```python
from build123d import *

# Parameters (mm, degrees)
SKETCH_1_R      = 1.65
EXTRUDE_1_DEPTH = 2
EXTRUDE_3_DEPTH = 23.5
SKETCH_3_R      = 1.5
EXTRUDE_4_DEPTH = 2
FILLET_1_R      = 1


with BuildPart() as part:
    # 草图1 → 凸台-拉伸1 (new body)
    # profile 1 of 2: a face of its own
    with BuildSketch(Plane(origin=(0, 0, 0), x_dir=(1, 0, 0), z_dir=(0, 1, 0))):
        with BuildLine():
            ThreePointArc((0, 1.5), (0.439339828, 0.439339828), (1.5, 0))
            Line((1.5, 0), (26.5, 0))
            ThreePointArc((26.5, 0), (27.560660172, 0.439339828), (28, 1.5))
            Line((28, 1.5), (28, 14))
            ThreePointArc((28, 14), (27.225183212, 18.592878075), (24.986495855, 22.677379145))
            ThreePointArc((24.986495855, 22.677379145), (22.833273811, 22.833273811), (22.677379145, 24.986495855))
            ThreePointArc((22.677379145, 24.986495855), (18.592878075, 27.225183212), (14, 28))
            Line((14, 28), (1.5, 28))
            ThreePointArc((1.5, 28), (0.439339828, 27.560660172), (0, 26.5))
            Line((0, 26.5), (0, 1.5))
        make_face()
        with Locations(Location((4, 4, 0), (0, 0, 270))):
            Circle(SKETCH_1_R, mode=Mode.SUBTRACT)
        with Locations(Location((24, 4, 0), (0, 0, 270))):
            Circle(SKETCH_1_R, mode=Mode.SUBTRACT)
        with Locations(Location((4, 24, 0), (0, 0, 270))):
            Circle(SKETCH_1_R, mode=Mode.SUBTRACT)
        with BuildLine():
            Line((18.75, 8.8), (9.25, 8.8))
            ThreePointArc((9.25, 8.8), (8.189339828, 9.239339828), (7.75, 10.3))
            Line((7.75, 10.3), (7.75, 17.7))
            ThreePointArc((7.75, 17.7), (8.189339828, 18.760660172), (9.25, 19.2))
            Line((9.25, 19.2), (18.75, 19.2))
            ThreePointArc((18.75, 19.2), (19.810660172, 18.760660172), (20.25, 17.7))
            Line((20.25, 17.7), (20.25, 10.3))
            ThreePointArc((20.25, 10.3), (19.810660172, 9.239339828), (18.75, 8.8))
        make_face(mode=Mode.SUBTRACT)
    # profile 2 of 2: a face of its own
    with BuildSketch(Plane(origin=(0, 0, 0), x_dir=(1, 0, 0), z_dir=(0, 1, 0))):
        with BuildLine():
            ThreePointArc((22.677379145, 24.986495855), (22.833273811, 22.833273811), (24.986495855, 22.677379145))
            ThreePointArc((24.986495855, 22.677379145), (23.899494937, 23.899494937), (22.677379145, 24.986495855))
        make_face()
    extrude(amount=EXTRUDE_1_DEPTH)

    # 草图2 → 凸台-拉伸3 (add)
    with BuildSketch(Plane(origin=(0, 2, 0), x_dir=(1, 0, 0), z_dir=(0, 1, 0))):
        with BuildLine():
            Line((7.25, 21.2), (20.75, 21.2))
            ThreePointArc((20.75, 21.2), (21.810660172, 20.760660172), (22.25, 19.7))
            Line((22.25, 19.7), (22.25, 8.3))
            ThreePointArc((22.25, 8.3), (21.810660172, 7.239339828), (20.75, 6.8))
            Line((20.75, 6.8), (7.25, 6.8))
            ThreePointArc((7.25, 6.8), (6.189339828, 7.239339828), (5.75, 8.3))
            Line((5.75, 8.3), (5.75, 19.7))
            ThreePointArc((5.75, 19.7), (6.189339828, 20.760660172), (7.25, 21.2))
        make_face()
        with BuildLine():
            Line((9.25, 19.2), (18.75, 19.2))
            ThreePointArc((18.75, 19.2), (19.810660172, 18.760660172), (20.25, 17.7))
            Line((20.25, 17.7), (20.25, 10.3))
            ThreePointArc((20.25, 10.3), (19.810660172, 9.239339828), (18.75, 8.8))
            Line((18.75, 8.8), (9.25, 8.8))
            ThreePointArc((9.25, 8.8), (8.189339828, 9.239339828), (7.75, 10.3))
            Line((7.75, 10.3), (7.75, 17.7))
            ThreePointArc((7.75, 17.7), (8.189339828, 18.760660172), (9.25, 19.2))
        make_face(mode=Mode.SUBTRACT)
    extrude(amount=EXTRUDE_3_DEPTH)

    # 草图3 → 凸台-拉伸4 (add)
    with BuildSketch(Plane(origin=(0, 25.5, 0), x_dir=(1, 0, 0), z_dir=(0, 1, 0))):
        with BuildLine():
            Line((22.25, 8.3), (22.25, 19.7))
            ThreePointArc((22.25, 19.7), (21.810660172, 20.760660172), (20.75, 21.2))
            Line((20.75, 21.2), (7.25, 21.2))
            ThreePointArc((7.25, 21.2), (6.189339828, 20.760660172), (5.75, 19.7))
            Line((5.75, 19.7), (5.75, 8.3))
            ThreePointArc((5.75, 8.3), (6.189339828, 7.239339828), (7.25, 6.8))
            Line((7.25, 6.8), (20.75, 6.8))
            ThreePointArc((20.75, 6.8), (21.810660172, 7.239339828), (22.25, 8.3))
        make_face()
        with Locations(Location((10.25, 14, 0), (0, 0, 270))):
            Circle(SKETCH_3_R, mode=Mode.SUBTRACT)
        with Locations(Location((17.75, 14, 0), (0, 0, 90))):
            Circle(SKETCH_3_R, mode=Mode.SUBTRACT)
    extrude(amount=EXTRUDE_4_DEPTH)

    # 圆角1
    fillet_1_edges = [part.edges().sort_by_distance(p)[0] for p in [
        (5.75, 2, -14),
        (14, 2, -21.2),
        (22.25, 2, -14),
        (14, 2, -6.8),
        (6.189339828, 2, -7.239339828),
        (21.810660172, 2, -7.239339828),
        (21.810660172, 2, -20.760660172),
        (6.189339828, 2, -20.760660172),
    ]]
    fillet(fillet_1_edges, radius=FILLET_1_R)


solid = part.part
```
Verification items for the finished model (mm, model axes). A direction names the side the tool comes from. Round coordinates to 2 decimals unless told otherwise and drop trailing zeros. Order: outer loops, then holes, each group sorted by start corner. A loop starts at its lowest first (then second) coordinate and runs counter-clockwise, first axis right, second up. Notation, with made-up numbers: (-39.75, -7) - (-25.75, -7) arc R16 ccw to (-25.75, 21) - close; hole circle Ø4 at (38.25, 66.5). An arc over 180 degrees is marked (long way). Use CSV: the item, a comma, the result in double quotes. Start each with the question number.
1) Section check C-C, the plane z = -3.25. Record the cut outline in (x, y).
2) Go/stop test with flat-tipped pins: P1, Ø7, axis at x = 13.5, y = 15, coming from the -Z side; P2, Ø9, axis at y = 20, z = -15, coming from the -X side; P3, Ø8, axis at y = 19, z = -3.5, coming from the -X side; P4, Ø2.5, axis at x = 4, z = -24, coming from the -Y side. Record where each tip stops, or that it passes through.
3) Mould release check, pull along Z, two halves, no side actions. Record for faces 1 (the flat face through (14, 27.5, -14)), 2 (the cylindrical face through (19.82, 12.57, -9.25)), 3 (the cylindrical face through (14.094, 2.285, -21.501)), 4 (the cylindrical face through (6.18, 15.08, -7.25)): +Z half, -Z half, draft (parallel to the pull), parting line (faces both ways), or undercut.
4) Section check A-A, the plane y = 16. Record the cut outline in (x, z), plus the area to 3 significant figures.
5) Thickness scan on L1, parallel to X at y = 0.6, z = -4; L2, parallel to X at y = 3.25, z = -14.75; L3, parallel to Z at x = 17.5, y = 13. Record the ranges inside material, lowest first.
6) Section check D-D, the plane z = -11.25. Record the cut outline in (x, y), plus the area to 3 significant figures.
7) Access from +Z, -Z, +X, -X, +Y, -Y to the whole of each face (thin tool, end or side, straight path). Record for faces 5 (the flat face through (14, 15, -6.8)), 6 (the cylindrical face through (21.8, 15.08, -7.23)), 7 (the flat face through (7.75, 13, -14)), 8 (the flat face through (5.75, 15, -14)).
8) Section check B-B, the plane x = 10.25. Record the cut outline in (y, z).
Answers:
1,outline,"(0, 0) - (2.53, 0) - (2.53, 2) - (0, 2) - close; (5.47, 0) - (22.53, 0) - (22.53, 2) - (5.47, 2) - close; (25.47, 0) - (28, 0) - (28, 2) - (25.47, 2) - close"
2,P1,"stops at z = -21.2"
2,P2,"stops at x = 5.75"
2,P3,"stops at x = 5.98"
2,P4,"passes through"
3,face 1,"draft"
3,face 2,"undercut"
3,face 3,"-Z half"
3,face 4,"+Z half"
4,outline,"(5.75, -19.7) arc R1.5 ccw to (7.25, -21.2) - (20.75, -21.2) arc R1.5 ccw to (22.25, -19.7) - (22.25, -8.3) arc R1.5 ccw to (20.75, -6.8) - (7.25, -6.8) arc R1.5 ccw to (5.75, -8.3) - close; hole (7.75, -17.7) arc R1.5 ccw to (9.25, -19.2) - (18.75, -19.2) arc R1.5 ccw to (20.25, -17.7) - (20.25, -10.3) arc R1.5 ccw to (18.75, -8.8) - (9.25, -8.8) arc R1.5 ccw to (7.75, -10.3) - close"
4,area,"108 mm²"
5,L1,"x = 0 to 2.35, 5.65 to 22.35, 25.65 to 28"
5,L2,"x = 5.75 to 7.75, 20.25 to 22.25"
5,L3,"z = -21.2 to -19.2, -8.8 to -6.8"
6,outline,"(0, 0) - (7.75, 0) - (7.75, 25.5) - (20.25, 25.5) - (20.25, 0) - (28, 0) - (28, 2) - (23.25, 2) arc R1 cw to (22.25, 3) - (22.25, 27.5) - (5.75, 27.5) - (5.75, 3) arc R1 cw to (4.75, 2) - (0, 2) - close"
6,area,"158 mm²"
7,face 5,"+Z, +X, -X, +Y"
7,face 6,"+Z, +X, +Y"
7,face 7,"-Y"
7,face 8,"+Z, -Z, -X, +Y"
8,outline,"(0, -28) - (2, -28) - (2, -22.2) arc R1 cw to (3, -21.2) - (27.5, -21.2) - (27.5, -15.5) - (25.5, -15.5) - (25.5, -19.2) - (0, -19.2) - close; (0, -8.8) - (25.5, -8.8) - (25.5, -12.5) - (27.5, -12.5) - (27.5, -6.8) - (3, -6.8) arc R1 cw to (2, -5.8) - (2, 0) - (0, 0) - close"
